from build123d import *

# Parameters (mm, degrees)
SKETCH21_R           = 10
BOSS_EXTRUDE20_DEPTH = 20
SKETCH24_W           = 10.018971209
SKETCH24_H           = 35.052940056
CUT_EXTRUDE10_DEPTH  = 20


with BuildPart() as part:
    # Sketch21 → Boss-Extrude20 (new body)
    with BuildSketch(Plane.XY):
        with BuildLine():
            Line((54.893048592, 39.689392996), (64.893048592, 39.689392996))
            Line((64.893048592, 39.689392996), (64.893048592, 84.689392996))
            Line((64.893048592, 84.689392996), (69.893048592, 84.689392996))
            ThreePointArc((69.893048592, 84.689392996), (75.770400953, 103.092850807), (91.226612731, 114.683193669))
            ThreePointArc((91.226612731, 114.683193669), (99.80843011, 136.069116434), (78.422507345, 144.650933813))
            ThreePointArc((78.422507345, 144.650933813), (54.7296652, 138.68102842), (31.036823055, 144.650933813))
            ThreePointArc((31.036823055, 144.650933813), (16.541386166, 133.13054606), (18.132679452, 114.683193669))
            ThreePointArc((18.132679452, 114.683193669), (39.470310291, 105.844857587), (48.308646374, 84.507226748))
            Line((48.308646374, 84.507226748), (54.893048592, 84.507226748))
            Line((54.893048592, 84.507226748), (54.893048592, 39.689392996))
        make_face()
        with Locations((84.824560038, 129.667063741)):
            Circle(SKETCH21_R, mode=Mode.SUBTRACT)
        with Locations((34.893048592, 127.050928279)):
            Circle(SKETCH21_R, mode=Mode.SUBTRACT)
    extrude(amount=BOSS_EXTRUDE20_DEPTH)

    # Sketch24 → Cut-Extrude10 (cut)
    with BuildSketch(Plane.ZY.offset(-54.893048592)):
        with Locations((10.125179514, 57.215863024)):
            Rectangle(SKETCH24_W, SKETCH24_H)
    extrude(amount=-CUT_EXTRUDE10_DEPTH, mode=Mode.SUBTRACT)


solid = part.part
Read the model definition and answer for the solid it produces. Units are mm, in the model's axes. A direction names the side the tool comes from. Give positions to 0.01 mm unless a question says otherwise; leave off trailing zeros. Write each loop counter-clockwise with the first axis right and the second up, starting at its lowest first coordinate (ties: lowest second). Pieces come first, ordered by that corner, then holes. Notation, with made-up numbers: (87, 75) - (118, 75) arc R6 cw to (118, 83) - close; hole circle Ø9 at (54, 10.25). An arc over 180 degrees is marked (long way). Use CSV: the item, a comma, the result in double quotes. Start each with the question number.
(1) Given P1, Ø8, axis at y = 107, z = 6, coming from the +X side; P2, Ø2.5, axis at x = 68.5, z = 9.5, coming from the -Y side; P3, Ø2, axis at y = 58, z = 2.5, coming from the -X side; P4, Ø18, axis at x = 84.82, y = 129.67, coming from the -Z side, each flat-ended and moving along its own axis, determine where each tip first touches the part or whether it passes through.
(2) Find section A-A (y = 63). Give the vertices of the cut face in (x, z), plus the area to 3 significant figures.
(3) Consider line 1 along X through (y, z) = (135.5, 6.75); line 2 along X through (y, z) = (126, 7); line 3 along Y through (x, z) = (93, 9.25). Determine where each line is inside the solid, lowest interval first.
(4) Find section C-C (z = 12.5). Give the vertices of the cut face in (x, y), plus the area to 3 significant figures.
(5) Find section D-D (x = 63). Give the vertices of the cut face in (y, z).
(6) For faces 4 (the flat face through (54.893, 67, 3)), 5 (the flat face through (60, 57, 15.135)), 6 (the flat face through (67, 84.689, 10)), determine the directions among +Z, -Z, +X, -X, +Y, -Y from which every point of the face is accessible in a straight line to the end or side of a thin tool.
(7) Find section B-B (x = 39). Give the vertices of the cut face in (y, z).
(8) Determine the mould class of faces 1 (the flat face through (58, 117, 20)), 2 (the cylindrical face through (82.657, 119.905, 9.86)), 3 (the cylindrical face through (16.65, 133.38, 9.86)) for opening direction X: +X half, -X half, draft (parallel to the pull), parting line (faces both ways), or undercut.
Findings below:
1,P1,"x = 83.87"
1,P2,"y = 84.69"
1,P3,"x = 54.89"
1,P4,"through"
2,outline,"(54.89, 0) - (64.89, 0) - (64.89, 5.12) - (54.89, 5.12) - close; (54.89, 15.13) - (64.89, 15.13) - (64.89, 20) - (54.89, 20) - close"
2,area,"99.8 mm2"
3,line 1,"17.76 to 29.54, 40.24 to 76.7, 92.95 to 100.04"
3,line 2,"14.96 to 24.95, 44.84 to 75.52, 94.13 to 100.7"
3,line 3,"115.57 to 123.91, 135.43 to 143.76"
4,outline,"(18.13, 114.68) arc R30.18 cw to (48.31, 84.51) - (54.89, 84.51) - (54.89, 74.74) - (64.89, 74.74) - (64.89, 84.69) - (69.89, 84.69) arc R31.75 cw to (91.23, 114.68) arc R16.29 ccw to (78.42, 144.65) arc R50 cw to (31.04, 144.65) arc R19.57 ccw to start; hole circle Ø20 at (34.89, 127.05); hole circle Ø20 at (84.82, 129.67)"
4,area,"2,720 mm2"
5,outline,"(39.69, 0) - (139.37, 0) - (139.37, 20) - (39.69, 20) - (39.69, 15.13) - (74.74, 15.13) - (74.74, 5.12) - (39.69, 5.12) - close"
6,face 4,"+Z, -Z, -X, -Y"
6,face 5,"+X, -X, -Y"
6,face 6,"+Z, -Z, +X, -Y"
7,outline,"(106.31, 0) - (117.93, 0) - (117.93, 20) - (106.31, 20) - close; (136.17, 0) - (141.22, 0) - (141.22, 20) - (136.17, 20) - close"
8,face 1,"draft"
8,face 2,"undercut"
8,face 3,"-X half"
